Part print with two shaded views. Sizes in mm from the minimum x, y, z corner. A direction names the side the tool comes from. Give positions to 0.01 mm unless a question says otherwise; leave off trailing zeros. Order: outer loops, then holes, each group sorted by start corner. A loop starts at its lowest first (then second) coordinate and runs counter-clockwise, first axis right, second up.
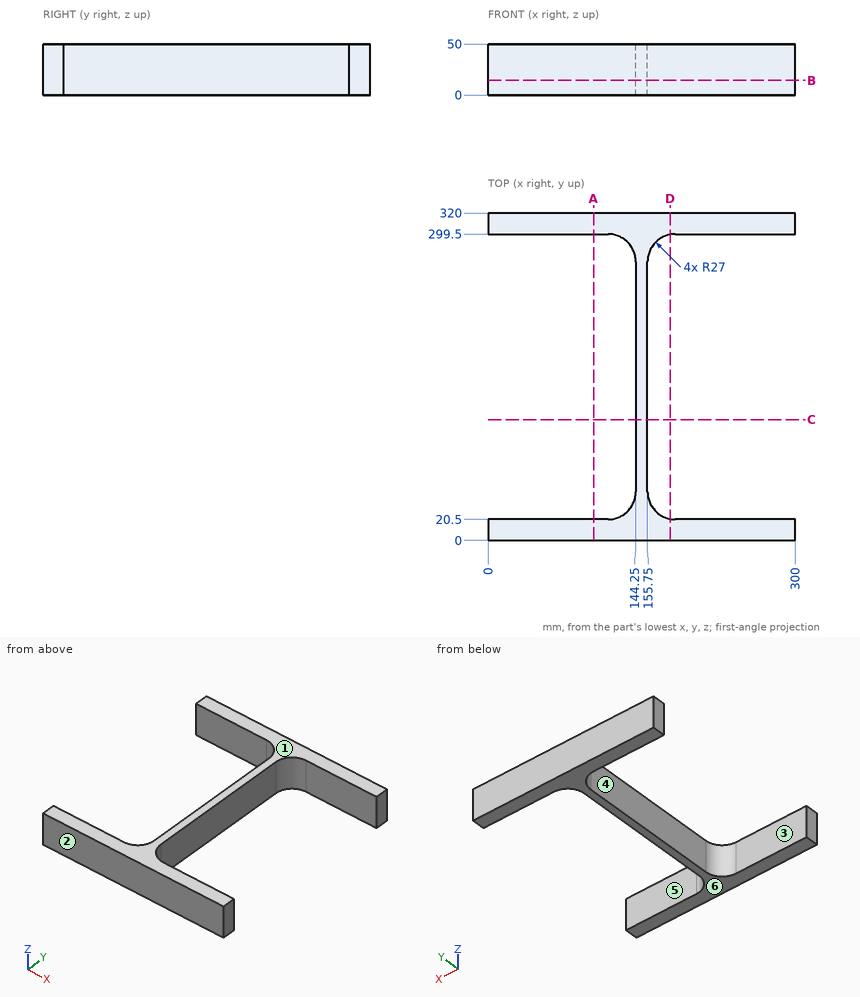
Item 1: Slice it at D-D (x = 178). Give the cut face in (y, z).
Item 2: Slice it at C-C (y = 118). Give the cut face in (x, z).
Item 3: Drop flat-ended pins along their axis: pin 1 Ø1 at (y, z) = (268.5, 41) entering from +X; pin 2 Ø6 at (y, z) = (73, 36.5) entering from -X; pin 3 Ø10 at (y, z) = (44, 33.5) entering from -X. Give the stop position or say it passes through.
Item 4: Slice it at B-B (z = 14.5). Give the cut face in (x, y).
Item 5: Slice it at A-A (x = 103). Give the cut face in (y, z).
Item 6: Wall check: L1, parallel to Y at x = 263, z = 13.5; L2, parallel to X at y = 245, z = 13.5; L3, parallel to Y at x = 165, z = 38.5. Give the ranges that are in metal, low to high.
Item 7: Tool access for the marked faces 4, 5 and 6: list every direction of +Z, -Z, +X, -X, +Y, -Y with a clear straight run to the whole face (end or side of a thin tool).
Item 8: Two-plate mould, pull along Y, no slides. Class the marked faces 1, 2 and 3: released by +Y, released by -Y, zero draft, split by the parting line, or undercut.
A:
1. outline: (0, 0) - (20.92, 0) - (20.92, 50) - (0, 50) - close; (299.08, 0) - (320, 0) - (320, 50) - (299.08, 50) - close
2. outline: (144.25, 0) - (155.75, 0) - (155.75, 50) - (144.25, 50) - close
3. pin 1: stops at x = 155.75
3. pin 2: stops at x = 144.25
3. pin 3: stops at x = 142.88
4. outline: (0, 0) - (300, 0) - (300, 20.5) - (182.75, 20.5) arc R27 cw to (155.75, 47.5) - (155.75, 272.5) arc R27 cw to (182.75, 299.5) - (300, 299.5) - (300, 320) - (0, 320) - (0, 299.5) - (117.25, 299.5) arc R27 cw to (144.25, 272.5) - (144.25, 47.5) arc R27 cw to (117.25, 20.5) - (0, 20.5) - close
5. outline: (0, 0) - (20.5, 0) - (20.5, 50) - (0, 50) - close; (299.5, 0) - (320, 0) - (320, 50) - (299.5, 50) - close
6. L1: y = 0 to 20.5, 299.5 to 320
6. L2: x = 144.25 to 155.75
6. L3: y = 0 to 27.15, 292.85 to 320
7. face 4: +Z, -Z, -X
7. face 5: +Z, -Z, +X
7. face 6: -Z, +X, -X, +Y, -Y
8. face 1: zero draft
8. face 2: released by -Y
8. face 3: undercut
